Can you work these out from the model? Positions are in its coordinate system, mm. A direction names the side the tool comes from. Round coordinates to 2 decimals unless told otherwise and drop trailing zeros. Loops run counter-clockwise (first coordinate to the right, second up) from the corner with the lowest first, then second, coordinate; pieces in that order, holes last.
(1) I want a section at A-A on z = -81.5. Write out the boundary of the cut face in (x, y).
(2) I want a section at B-B on y = 26.5. Write out the boundary of the cut face in (x, z).
(3) I want a section at C-C on z = -53.5. Write out the boundary of the cut face in (x, y).
(4) Will these pins go through, and if not, where does the flat tip stop? pin 1 Ø4 at (y, z) = (-7, -75.5) entering from +X; pin 2 Ø4 at (x, y) = (-6, -24) entering from +Z; pin 3 Ø0.8 at (x, y) = (4, -38.5) entering from -Z.
(5) If I drill on line 1 along X through (y, z) = (-40.5, -85); line 2 along Y through (x, z) = (2.75, -74.5); line 3 along Z through (x, y) = (-5, 9), over which ranges is the centre line in solid material (lowest first)?
(6) Thinking about a two-plate mould opening in Y: for faces 4 (the face through (-0.126, -11.047, -59.345)), 5 (the face through (8.26, 34.756, -55.487)), 6 (the face through (10.5, -7, -66)), which applies, released by +Y, released by -Y, zero draft, split by the parting line, or undercut?
(7) Which directions (+Z, -Z, +X, -X, +Y, -Y) give clear straight access to the entire face, cutting with the end or side of a thin tool? Please do faces 1 (the face through (-8.26, 37.75, -61.946)), 2 (the face through (0.126, -44.877, -93.013)), 3 (the face through (8.26, 59.897, -52.481)).
(8) I want a section at D-D on y = -19.5. Write out the boundary of the cut face in (x, z).
from build123d import *

# Parameters (mm, degrees)
BOSS_EXTRUDE1_DEPTH = 9
CUT_EXTRUDE1_DEPTH  = 25
BOSS_EXTRUDE2_DEPTH = 18
LPATTERN1_COUNT     = 5
LPATTERN1_PITCH     = 5
FILLET2_R           = 5
FILLET3_R           = 8
SKETCH4_R           = 1.5
CUT_EXTRUDE2_DEPTH  = 18
SKETCH6_W           = 6
SKETCH6_H           = 18.02956864
CUT_EXTRUDE3_DEPTH  = 8
SKETCH7_R           = 1.75
BOSS_EXTRUDE3_DEPTH = 1.5
CUT_EXTRUDE8_DEPTH  = 1.5


with BuildPart() as part:
    # Sketch1 → Boss-Extrude1 (new, symmetric)
    with BuildSketch(Plane(origin=(0, 0, 0), x_dir=(0, 0, -1), z_dir=(1, 0, 0))):
        with BuildLine():
            Line((90.984883898, -2.862650195), (95.574427473, 6.021948264))
            ThreePointArc((95.574427473, 6.021948264), (92.997394543, 14.106433484), (84.912909322, 11.529400554))
            Line((84.912909322, 11.529400554), (79.647841616, 1.337098931))
            Line((79.647841616, 1.337098931), (72.241979914, 3.428014696))
            Line((72.241979914, 3.428014696), (62.847901181, 0))
            Line((62.847901181, 0), (58.150861814, -1.714007348))
            Line((58.150861814, -1.714007348), (58.150861814, -11.714007348))
            Line((58.150861814, -11.714007348), (69.700839811, -17.680413995))
            Line((69.700839811, -17.680413995), (79.984883898, -45.862650195))
            Line((79.984883898, -45.862650195), (79.984883898, -52.862650195))
            Line((79.984883898, -52.862650195), (90.984883898, -52.862650195))
            Line((90.984883898, -52.862650195), (90.984883898, -2.862650195))
        make_face()
        Polygon((72.241979914, 3.428014696), (62.847901181, 0), (38.851798311, 65.758551133), (61.529389306, 73.615195879), align=None)
    extrude(amount=BOSS_EXTRUDE1_DEPTH, both=True)

    # Sketch2 → Cut-Extrude1 (cut)
    with BuildSketch(Plane(origin=(9, 0, 0), x_dir=(0, 0, -1), z_dir=(1, 0, 0))):
        Polygon((88.284883898, -45.862650195), (88.284883898, -20.862650195), (73.284883898, -20.862650195), align=None)
    extrude(amount=-CUT_EXTRUDE1_DEPTH, mode=Mode.SUBTRACT)

    # Sketch3 → Boss-Extrude2 (add)
    with BuildSketch(Plane(origin=(9, 0, 0), x_dir=(0, 0, -1), z_dir=(1, 0, 0))):
        Polygon((94.984883898, -45.862650195), (90.984883898, -45.862650195), (90.984883898, -47.862650195), align=None)
        Polygon((90.984883898, -43.862650195), (90.984883898, -45.862650195), (94.984883898, -45.862650195), align=None)
    boss_extrude2 = extrude(amount=-BOSS_EXTRUDE2_DEPTH)

    # LPattern1: Boss-Extrude2 ×5
    with Locations(*[(0, i * LPATTERN1_PITCH, 0) for i in range(1, LPATTERN1_COUNT)]):
        add(boss_extrude2)

    # Fillet2
    fillet2_edges = [part.edges().sort_by_distance(p)[0] for p in [
        (0, 65.758551133, -38.851798311),
        (0, 73.615195879, -61.529389306),
    ]]
    fillet(fillet2_edges, radius=FILLET2_R)

    # Fillet3
    # the kernel refuses this fillet: 8 mm, written as the material it takes off along each edge
    with BuildSketch(Plane(origin=(-21.179405631, -11.714007348, -58.150861814), x_dir=(0, 1, 0), z_dir=(1, 0, 0))) as fillet3_piece_1:
        with BuildLine():
            CenterArc((FILLET3_R * 0.608970281556, -FILLET3_R), FILLET3_R, 90, 62.680345336)
            Line((-FILLET3_R * 0.279489564314, -FILLET3_R * 0.541045642491), (-FILLET3_R * 0.297258761231, -FILLET3_R * 0.531866555341))
            Line((-FILLET3_R * 0.297258761231, -FILLET3_R * 0.531866555341), (-FILLET3_R * 0.0121794056311, FILLET3_R * 0.02))
            Line((-FILLET3_R * 0.0121794056311, FILLET3_R * 0.02), (FILLET3_R * 0.608970281556, FILLET3_R * 0.02))
            Line((FILLET3_R * 0.608970281556, FILLET3_R * 0.02), (FILLET3_R * 0.608970281556, 0))
        make_face()
    extrude(amount=42.358811262, mode=Mode.SUBTRACT)
    with BuildSketch(Plane(origin=(-22.930780243, -1.714007348, -58.150861814), x_dir=(0, 0.34280146956229973, -0.9394078733254942), z_dir=(1, 0, 0))) as fillet3_piece_2:
        with BuildLine():
            CenterArc((5.605066211, -7.977085613), FILLET3_R, 94.33760972, 65.614743341)
            Line((-1.910196776, -5.234673857), (-2.060502036, -5.179825622))
            Line((-2.060502036, -5.179825622), (-0.15030526, 0.054848235))
            Line((-0.15030526, 0.054848235), (0, 0.16))
            ThreePointArc((0, 0.16), (2.5, 0.16), (4.987898676, 0.159541712))
            Line((4.987898676, 0.159541712), (5, 0))
        make_face()
    extrude(amount=45.861560486, mode=Mode.SUBTRACT)

    # Sketch4 → Cut-Extrude2 (cut)
    with BuildSketch(Plane(origin=(9, 0, 0), x_dir=(0, 0, -1), z_dir=(1, 0, 0))):
        with Locations((45.291168566, 62.697901722)):
            Circle(SKETCH4_R)
    extrude(amount=-CUT_EXTRUDE2_DEPTH, mode=Mode.SUBTRACT)

    # Sketch6 → Cut-Extrude3 (cut)
    with BuildSketch(Plane(origin=(0, 20.368113495, -55.816464867), x_dir=(1, 0, 0), z_dir=(0, -0.342801469564146, 0.9394078733248205))):
        with Locations((-3, -58.877510112)):
            Rectangle(SKETCH6_W, SKETCH6_H)
        with Locations((3, -58.877510112)):
            Rectangle(SKETCH6_W, SKETCH6_H)
    extrude(amount=-CUT_EXTRUDE3_DEPTH, mode=Mode.SUBTRACT)

    # Sketch7 → Boss-Extrude3 (add)
    with BuildSketch(Plane(origin=(9, 0, 0), x_dir=(0, 0, -1), z_dir=(1, 0, 0))):
        with Locations((90.243668397, 8.775674409)):
            Circle(SKETCH7_R)
        with Locations((66.150861814, -6.842245095)):
            Circle(SKETCH7_R)
    boss_extrude3 = extrude(amount=BOSS_EXTRUDE3_DEPTH)

    # Sketch9 → Cut-Extrude8 (cut)
    with BuildSketch(Plane(origin=(9, 0, 0), x_dir=(0, 0, -1), z_dir=(1, 0, 0))):
        with BuildLine():
            Line((58.440866419, 60.71212793), (65.549781573, 14.135652246))
            ThreePointArc((65.549781573, 14.135652246), (65.554544576, 13.869334092), (65.488833832, 13.611205938))
            Line((65.488833832, 13.611205938), (65.263485326, 13.051639762))
            ThreePointArc((65.263485326, 13.051639762), (64.319406176, 12.425340234), (63.396473347, 13.082403042))
            Line((63.396473347, 13.082403042), (47.353872306, 57.045300124))
            ThreePointArc((47.353872306, 57.045300124), (47.390108621, 57.817381382), (47.965919982, 58.333001219))
            Line((47.965919982, 58.333001219), (57.124954374, 61.506145996))
            ThreePointArc((57.124954374, 61.506145996), (57.968947683, 61.417453255), (58.440866419, 60.71212793))
        make_face()
    cut_extrude8 = extrude(amount=-CUT_EXTRUDE8_DEPTH, mode=Mode.SUBTRACT)

    # Mirror1: Boss-Extrude3, Cut-Extrude8 across plane
    add(boss_extrude3.mirror(Plane(origin=(0, 0, 0), x_dir=(0, 0, 1), z_dir=(1, 0, 0))))
    add(cut_extrude8.mirror(Plane(origin=(0, 0, 0), x_dir=(0, 0, 1), z_dir=(1, 0, 0))), mode=Mode.SUBTRACT)


solid = part.part
Filled sheet:
1. outline: (-9, -52.86) - (9, -52.86) - (9, -34.55) - (6, -34.55) - (6, -42.53) - (-6, -42.53) - (-6, -34.55) - (-9, -34.55) - close; (-9, -20.86) - (9, -20.86) - (9, 4.92) - (-9, 4.92) - close
2. outline: (-9, -68.72) - (9, -68.72) - (9, -63.66) - (7.5, -63.66) - (7.5, -58.5) - (9, -58.5) - (9, -53.18) - (-9, -53.18) - (-9, -58.5) - (-7.5, -58.5) - (-7.5, -63.66) - (-9, -63.66) - close
3. outline: (-9, 25.62) - (9, 25.62) - (9, 40.2) - (7.5, 40.2) - (7.5, 60.25) - (9, 60.25) - (9, 70.83) - (-9, 70.83) - (-9, 60.25) - (-7.5, 60.25) - (-7.5, 40.2) - (-9, 40.2) - close
4. pin 1: stops at x = 9
4. pin 2: stops at z = -71.28
4. pin 3: stops at z = -91.06
5. line 1: x = -9 to -6, 6 to 9
5. line 2: y = -25.89 to -22.89, -20.86 to 2.79
5. line 3: z = -96.24 to -83.61, -71.39 to -59.56
6. face 4: released by -Y
6. face 5: undercut
6. face 6: zero draft
7. face 1: -X
7. face 2: -Z, +X, -X
7. face 3: +X
8. outline: (-9, -90.98) - (9, -90.98) - (9, -70.36) - (-9, -70.36) - close
